For this review, use the dimensioned drawing (mm, ordinates from the lowest corner) and the shaded views. Give positions to 0.01 mm unless a question says otherwise; leave off trailing zeros. Write each loop counter-clockwise with the first axis right and the second up, starting at its lowest first coordinate (ties: lowest second). Pieces come first, ordered by that corner, then holes. Notation, with made-up numbers: M 19,27 L 29,27 A22 cw 29,49 Z; hole C 88.25,-13.5 d1. An arc over 180 degrees is marked long. Answer in a Markdown table with one row per item.
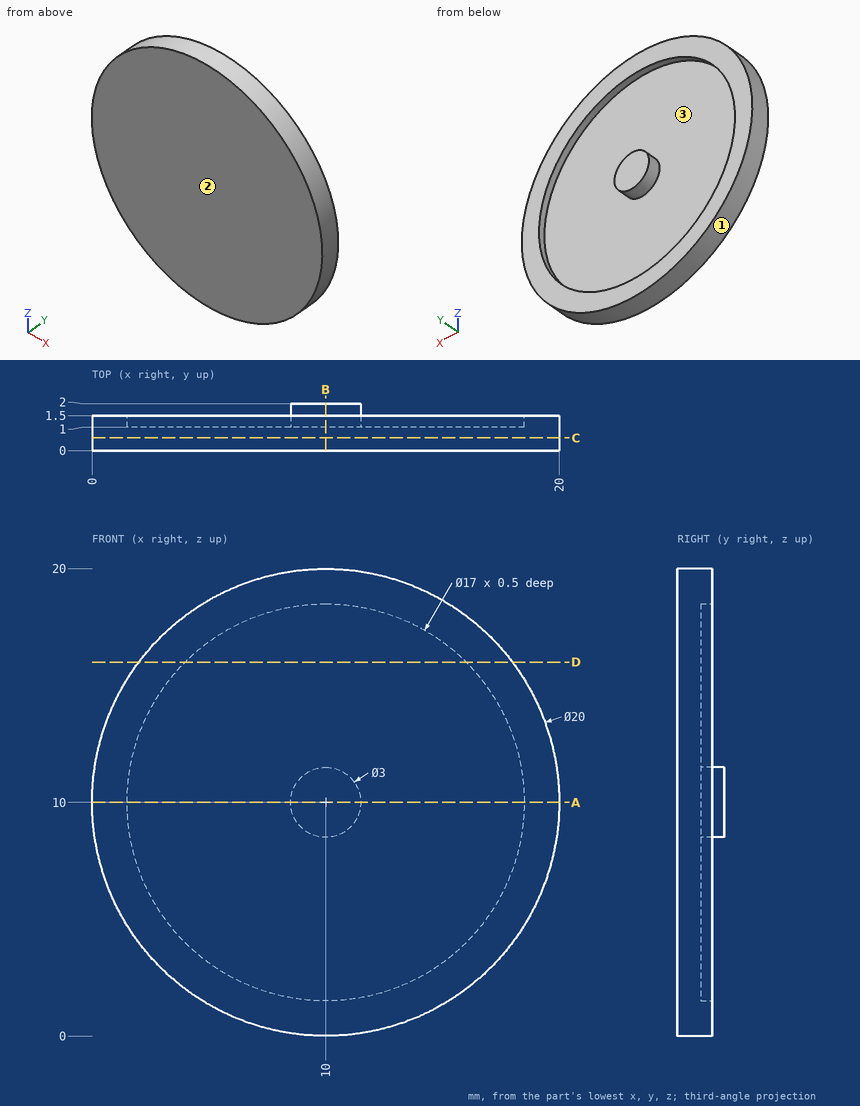
1) The part is to be moulded in two halves that separate along Z. For the marked faces 1, 2 and 3, say which applies: released by +Z, released by -Z, zero draft, split by the parting line, or undercut.
Geometry says:
| item | result |
|---|---|
| face 1 | split by the parting line |
| face 2 | zero draft |
| face 3 | undercut |
2) Add section B-B (x = 10). Write out the cut boundary in (y, z), and give its area (3 significant figures).
Geometry says:
| item | result |
|---|---|
| outline | M 0,0 L 1.5,0 L 1.5,1.5 L 1,1.5 L 1,8.5 L 2,8.5 L 2,11.5 L 1,11.5 L 1,18.5 L 1.5,18.5 L 1.5,20 L 0,20 Z |
| area | 24.5 mm^2 |
3) Add section D-D (z = 16). Write out the cut boundary in (x, y), and give its area (3 significant figures).
Geometry says:
| item | result |
|---|---|
| outline | M 2,0 L 18,0 L 18,1.5 L 16.02,1.5 L 16.02,1 L 3.98,1 L 3.98,1.5 L 2,1.5 Z |
| area | 18.0 mm^2 |
4) Add section C-C (y = 0.55). Write out the cut boundary in (x, z), and give its area (3 significant figures).
Geometry says:
| item | result |
|---|---|
| outline | C 10,10 d20 |
| area | 314 mm^2 |
5) Add section A-A (z = 10). Write out the cut boundary in (x, y), and give its area (3 significant figures).
Geometry says:
| item | result |
|---|---|
| outline | M 0,0 L 20,0 L 20,1.5 L 18.5,1.5 L 18.5,1 L 11.5,1 L 11.5,2 L 8.5,2 L 8.5,1 L 1.5,1 L 1.5,1.5 L 0,1.5 Z |
| area | 24.5 mm^2 |
6) Insertion check: P1, Ø8, axis at x = 5, z = 7, coming from the +Y side; P2, Ø1, axis at y = 1, z = 14.5, coming from the +X side. Each pin has a flat end and moves straight along its axis. Give the tip position at first contact, or say it passes through.
Geometry says:
| item | result |
|---|---|
| P1 | y = 1.5 |
| P2 | x = 19.17 |
7) To check wall thickness, follow probe 1 along X at (y, z) = (1.3, 10); probe 2 along Y at (x, z) = (2.5, 13); probe 3 along X at (y, z) = (0.7, 10). State the ranges of each line that lie inside material, in increasing order. Write a range as [from, to].
Geometry says:
| item | result |
|---|---|
| probe 1 | [0, 1.5], [8.5, 11.5], [18.5, 20] |
| probe 2 | [0, 1] |
| probe 3 | [0, 20] |
